from build123d import *

# Parameters (mm, degrees)
SKETCH1_W           = 70
SKETCH1_H           = 70
SKETCH1_R           = 1.65
BOSS_EXTRUDE1_DEPTH = 6.35
CUT_EXTRUDE1_REACH  = 51.903
SKETCH2_R           = 1.1
CUT_EXTRUDE2_REACH  = 51.903
SKETCH3_R           = 9.65
CUT_EXTRUDE3_REACH  = 51.903
SKETCH4_R           = 2.1
SKETCH5_R           = 4.5
CUT_EXTRUDE4_DEPTH  = 2.5


with BuildPart() as part:
    # Sketch1 → Boss-Extrude1 (new body)
    with BuildSketch(Plane(origin=(0, 0, 0), x_dir=(1, 0, 0), z_dir=(0, 1, 0))):
        Rectangle(SKETCH1_W, SKETCH1_H)
        with Locations(Location((0, 13, 0), (0, 0, 270))):
            Circle(SKETCH1_R, mode=Mode.SUBTRACT)
        with Locations(Location((13, 0, 0), (0, 0, 270))):
            Circle(SKETCH1_R, mode=Mode.SUBTRACT)
        with Locations(Location((0, -13, 0), (0, 0, 270))):
            Circle(SKETCH1_R, mode=Mode.SUBTRACT)
        with Locations(Location((-13, 0, 0), (0, 0, 270))):
            Circle(SKETCH1_R, mode=Mode.SUBTRACT)
    extrude(amount=BOSS_EXTRUDE1_DEPTH)

    # Sketch2 → Cut-Extrude1 (cut, up to next)
    with BuildSketch(Plane(origin=(0, 6.35, 0), x_dir=(1, 0, 0), z_dir=(0, 1, 0)), mode=Mode.PRIVATE) as cut_extrude1_sk1:
        with Locations(Location((16.375, 28, 0), (0, 0, 270))):
            Circle(SKETCH2_R)
    cut_extrude1_tool1 = extrude(cut_extrude1_sk1.sketch, amount=-CUT_EXTRUDE1_REACH, mode=Mode.PRIVATE) & part.part
    # Sketch2 → Cut-Extrude1 (cut, up to next)
    with BuildSketch(Plane(origin=(0, 6.35, 0), x_dir=(1, 0, 0), z_dir=(0, 1, 0)), mode=Mode.PRIVATE) as cut_extrude1_sk2:
        with Locations(Location((28.375, 28, 0), (0, 0, 270))):
            Circle(SKETCH2_R)
    cut_extrude1_tool2 = extrude(cut_extrude1_sk2.sketch, amount=-CUT_EXTRUDE1_REACH, mode=Mode.PRIVATE) & part.part
    # Sketch2 → Cut-Extrude1 (cut, up to next)
    with BuildSketch(Plane(origin=(0, 6.35, 0), x_dir=(1, 0, 0), z_dir=(0, 1, 0)), mode=Mode.PRIVATE) as cut_extrude1_sk3:
        with Locations(Location((28.375, 20, 0), (0, 0, 270))):
            Circle(SKETCH2_R)
    cut_extrude1_tool3 = extrude(cut_extrude1_sk3.sketch, amount=-CUT_EXTRUDE1_REACH, mode=Mode.PRIVATE) & part.part
    # Sketch2 → Cut-Extrude1 (cut, up to next)
    with BuildSketch(Plane(origin=(0, 6.35, 0), x_dir=(1, 0, 0), z_dir=(0, 1, 0)), mode=Mode.PRIVATE) as cut_extrude1_sk4:
        with Locations(Location((-28.375, 20, 0), (0, 0, 270))):
            Circle(SKETCH2_R)
    cut_extrude1_tool4 = extrude(cut_extrude1_sk4.sketch, amount=-CUT_EXTRUDE1_REACH, mode=Mode.PRIVATE) & part.part
    # Sketch2 → Cut-Extrude1 (cut, up to next)
    with BuildSketch(Plane(origin=(0, 6.35, 0), x_dir=(1, 0, 0), z_dir=(0, 1, 0)), mode=Mode.PRIVATE) as cut_extrude1_sk5:
        with Locations(Location((-28.375, 28, 0), (0, 0, 270))):
            Circle(SKETCH2_R)
    cut_extrude1_tool5 = extrude(cut_extrude1_sk5.sketch, amount=-CUT_EXTRUDE1_REACH, mode=Mode.PRIVATE) & part.part
    # Sketch2 → Cut-Extrude1 (cut, up to next)
    with BuildSketch(Plane(origin=(0, 6.35, 0), x_dir=(1, 0, 0), z_dir=(0, 1, 0)), mode=Mode.PRIVATE) as cut_extrude1_sk6:
        with Locations(Location((-16.375, 28, 0), (0, 0, 270))):
            Circle(SKETCH2_R)
    cut_extrude1_tool6 = extrude(cut_extrude1_sk6.sketch, amount=-CUT_EXTRUDE1_REACH, mode=Mode.PRIVATE) & part.part
    # Sketch2 → Cut-Extrude1 (cut, up to next)
    with BuildSketch(Plane(origin=(0, 6.35, 0), x_dir=(1, 0, 0), z_dir=(0, 1, 0)), mode=Mode.PRIVATE) as cut_extrude1_sk7:
        with Locations(Location((28.375, -20, 0), (0, 0, 270))):
            Circle(SKETCH2_R)
    cut_extrude1_tool7 = extrude(cut_extrude1_sk7.sketch, amount=-CUT_EXTRUDE1_REACH, mode=Mode.PRIVATE) & part.part
    # Sketch2 → Cut-Extrude1 (cut, up to next)
    with BuildSketch(Plane(origin=(0, 6.35, 0), x_dir=(1, 0, 0), z_dir=(0, 1, 0)), mode=Mode.PRIVATE) as cut_extrude1_sk8:
        with Locations(Location((28.375, -28, 0), (0, 0, 270))):
            Circle(SKETCH2_R)
    cut_extrude1_tool8 = extrude(cut_extrude1_sk8.sketch, amount=-CUT_EXTRUDE1_REACH, mode=Mode.PRIVATE) & part.part
    # Sketch2 → Cut-Extrude1 (cut, up to next)
    with BuildSketch(Plane(origin=(0, 6.35, 0), x_dir=(1, 0, 0), z_dir=(0, 1, 0)), mode=Mode.PRIVATE) as cut_extrude1_sk9:
        with Locations(Location((16.375, -28, 0), (0, 0, 270))):
            Circle(SKETCH2_R)
    cut_extrude1_tool9 = extrude(cut_extrude1_sk9.sketch, amount=-CUT_EXTRUDE1_REACH, mode=Mode.PRIVATE) & part.part
    # Sketch2 → Cut-Extrude1 (cut, up to next)
    with BuildSketch(Plane(origin=(0, 6.35, 0), x_dir=(1, 0, 0), z_dir=(0, 1, 0)), mode=Mode.PRIVATE) as cut_extrude1_sk10:
        with Locations(Location((-16.375, -28, 0), (0, 0, 270))):
            Circle(SKETCH2_R)
    cut_extrude1_tool10 = extrude(cut_extrude1_sk10.sketch, amount=-CUT_EXTRUDE1_REACH, mode=Mode.PRIVATE) & part.part
    # Sketch2 → Cut-Extrude1 (cut, up to next)
    with BuildSketch(Plane(origin=(0, 6.35, 0), x_dir=(1, 0, 0), z_dir=(0, 1, 0)), mode=Mode.PRIVATE) as cut_extrude1_sk11:
        with Locations(Location((-28.375, -20, 0), (0, 0, 270))):
            Circle(SKETCH2_R)
    cut_extrude1_tool11 = extrude(cut_extrude1_sk11.sketch, amount=-CUT_EXTRUDE1_REACH, mode=Mode.PRIVATE) & part.part
    # Sketch2 → Cut-Extrude1 (cut, up to next)
    with BuildSketch(Plane(origin=(0, 6.35, 0), x_dir=(1, 0, 0), z_dir=(0, 1, 0)), mode=Mode.PRIVATE) as cut_extrude1_sk12:
        with Locations(Location((-28.375, -28, 0), (0, 0, 270))):
            Circle(SKETCH2_R)
    cut_extrude1_tool12 = extrude(cut_extrude1_sk12.sketch, amount=-CUT_EXTRUDE1_REACH, mode=Mode.PRIVATE) & part.part
    add(cut_extrude1_tool1.solids().sort_by_distance((16.375, 6.35, -28))[0], mode=Mode.SUBTRACT)
    add(cut_extrude1_tool2.solids().sort_by_distance((28.375, 6.35, -28))[0], mode=Mode.SUBTRACT)
    add(cut_extrude1_tool3.solids().sort_by_distance((28.375, 6.35, -20))[0], mode=Mode.SUBTRACT)
    add(cut_extrude1_tool4.solids().sort_by_distance((-28.375, 6.35, -20))[0], mode=Mode.SUBTRACT)
    add(cut_extrude1_tool5.solids().sort_by_distance((-28.375, 6.35, -28))[0], mode=Mode.SUBTRACT)
    add(cut_extrude1_tool6.solids().sort_by_distance((-16.375, 6.35, -28))[0], mode=Mode.SUBTRACT)
    add(cut_extrude1_tool7.solids().sort_by_distance((28.375, 6.35, 20))[0], mode=Mode.SUBTRACT)
    add(cut_extrude1_tool8.solids().sort_by_distance((28.375, 6.35, 28))[0], mode=Mode.SUBTRACT)
    add(cut_extrude1_tool9.solids().sort_by_distance((16.375, 6.35, 28))[0], mode=Mode.SUBTRACT)
    add(cut_extrude1_tool10.solids().sort_by_distance((-16.375, 6.35, 28))[0], mode=Mode.SUBTRACT)
    add(cut_extrude1_tool11.solids().sort_by_distance((-28.375, 6.35, 20))[0], mode=Mode.SUBTRACT)
    add(cut_extrude1_tool12.solids().sort_by_distance((-28.375, 6.35, 28))[0], mode=Mode.SUBTRACT)

    # Sketch3 → Cut-Extrude2 (cut, up to next)
    with BuildSketch(Plane(origin=(0, 6.35, 0), x_dir=(1, 0, 0), z_dir=(0, 1, 0)), mode=Mode.PRIVATE) as cut_extrude2_sk1:
        with Locations(Location((0, 0, 0), (0, 0, 270))):
            Circle(SKETCH3_R)
    cut_extrude2_tool1 = extrude(cut_extrude2_sk1.sketch, amount=-CUT_EXTRUDE2_REACH, mode=Mode.PRIVATE) & part.part
    add(cut_extrude2_tool1.solids().sort_by_distance((0, 6.35, 0))[0], mode=Mode.SUBTRACT)

    # Sketch4 → Cut-Extrude3 (cut, up to next)
    with BuildSketch(Plane(origin=(0, 6.35, 0), x_dir=(1, 0, 0), z_dir=(0, 1, 0)), mode=Mode.PRIVATE) as cut_extrude3_sk1:
        with Locations(Location((0, 27.5, 0), (0, 0, 270))):
            Circle(SKETCH4_R)
    cut_extrude3_tool1 = extrude(cut_extrude3_sk1.sketch, amount=-CUT_EXTRUDE3_REACH, mode=Mode.PRIVATE) & part.part
    # Sketch4 → Cut-Extrude3 (cut, up to next)
    with BuildSketch(Plane(origin=(0, 6.35, 0), x_dir=(1, 0, 0), z_dir=(0, 1, 0)), mode=Mode.PRIVATE) as cut_extrude3_sk2:
        with Locations(Location((27.5, 0, 0), (0, 0, 270))):
            Circle(SKETCH4_R)
    cut_extrude3_tool2 = extrude(cut_extrude3_sk2.sketch, amount=-CUT_EXTRUDE3_REACH, mode=Mode.PRIVATE) & part.part
    # Sketch4 → Cut-Extrude3 (cut, up to next)
    with BuildSketch(Plane(origin=(0, 6.35, 0), x_dir=(1, 0, 0), z_dir=(0, 1, 0)), mode=Mode.PRIVATE) as cut_extrude3_sk3:
        with Locations(Location((0, -27.5, 0), (0, 0, 270))):
            Circle(SKETCH4_R)
    cut_extrude3_tool3 = extrude(cut_extrude3_sk3.sketch, amount=-CUT_EXTRUDE3_REACH, mode=Mode.PRIVATE) & part.part
    # Sketch4 → Cut-Extrude3 (cut, up to next)
    with BuildSketch(Plane(origin=(0, 6.35, 0), x_dir=(1, 0, 0), z_dir=(0, 1, 0)), mode=Mode.PRIVATE) as cut_extrude3_sk4:
        with Locations(Location((-27.5, 0, 0), (0, 0, 270))):
            Circle(SKETCH4_R)
    cut_extrude3_tool4 = extrude(cut_extrude3_sk4.sketch, amount=-CUT_EXTRUDE3_REACH, mode=Mode.PRIVATE) & part.part
    add(cut_extrude3_tool1.solids().sort_by_distance((0, 6.35, -27.5))[0], mode=Mode.SUBTRACT)
    add(cut_extrude3_tool2.solids().sort_by_distance((27.5, 6.35, 0))[0], mode=Mode.SUBTRACT)
    add(cut_extrude3_tool3.solids().sort_by_distance((0, 6.35, 27.5))[0], mode=Mode.SUBTRACT)
    add(cut_extrude3_tool4.solids().sort_by_distance((-27.5, 6.35, 0))[0], mode=Mode.SUBTRACT)

    # Sketch5 → Cut-Extrude4 (cut)
    with BuildSketch(Plane(origin=(0, 6.35, 0), x_dir=(1, 0, 0), z_dir=(0, 1, 0))):
        with Locations(Location((0, 27.5, 0), (0, 0, 270))):
            Circle(SKETCH5_R)
        with Locations(Location((27.5, 0, 0), (0, 0, 270))):
            Circle(SKETCH5_R)
        with Locations(Location((0, -27.5, 0), (0, 0, 270))):
            Circle(SKETCH5_R)
        with Locations(Location((-27.5, 0, 0), (0, 0, 270))):
            Circle(SKETCH5_R)
    extrude(amount=-CUT_EXTRUDE4_DEPTH, mode=Mode.SUBTRACT)


solid = part.part
Build history of the part. All positions in model axes, mm. A direction names the side the tool comes from. Round coordinates to 2 decimals unless told otherwise and drop trailing zeros. Loops run counter-clockwise (first coordinate to the right, second up) from the corner with the lowest first, then second, coordinate; pieces in that order, holes last. Notation, with made-up numbers: (68, 40.5) -> (93, 40.5) arc R10 ccw to (93, 48.5) -> close; hole circle Ø1 at (38, 2). An arc over 180 degrees is marked (long way). One line per item, written item: value. Start each with the question number.
Q1. Drop flat-ended pins along their axis: pin 1 Ø2.5 at (x, z) = (0, -13) entering from -Y; pin 2 Ø2.5 at (x, z) = (1, -27.5) entering from +Y. Give the stop position or say it passes through.
Q2. Cut at C-C on y = 2. Count the separate pieces of the cut face and the enclosed holes in it, plus the area to 3 significant figures.
Q3. Cut at B-B on z = -13. List the corners of the cut face in (x, y), plus the area to 3 significant figures.
Q4. Cut at D-D on z = -28. List the corners of the cut face in (x, y) (3 decimals).
Q5. 3-axis set-ups, long thin cutter, end or side, ignore diameter. For faces 1 (the face through (9.568, 3.219, -1.256)), 2 (the face through (29, 3.85, 2)): which of +Z, -Z, +X, -X, +Y, -Y reach the whole face in a straight line?
Q6. Two-plate mould, pull along Z, no slides. Class faces 3 (the face through (0, 3, 35)), 4 (the face through (-17.45, 3.22, -28.24)), 5 (the face through (35, 3, 0)): released by +Z, released by -Z, zero draft, split by the parting line, or undercut.
Q7. Probe line 1 along X through (y, z) = (4.25, 20) (3 decimals); line 2 along X through (y, z) = (4.5, -1); line 3 along X through (y, z) = (6, -2). List the from-to ranges inside material, lowest first.
Q8. Cut at A-A on z = 20. List the corners of the cut face in (x, y) (3 decimals).
Computed:
1. pin 1: through
1. pin 2: y = 3.85
2. separate pieces: 1
2. enclosed holes: 21
2. area: 4,470 mm²
3. outline: (-35, 0) -> (-1.65, 0) -> (-1.65, 6.35) -> (-35, 6.35) -> close; (1.65, 0) -> (35, 0) -> (35, 6.35) -> (1.65, 6.35) -> close
3. area: 424 mm²
4. outline: (-35, 0) -> (-29.475, 0) -> (-29.475, 6.35) -> (-35, 6.35) -> close; (-27.275, 0) -> (-17.475, 0) -> (-17.475, 6.35) -> (-27.275, 6.35) -> close; (-15.275, 0) -> (-2.04, 0) -> (-2.04, 3.85) -> (-4.472, 3.85) -> (-4.472, 6.35) -> (-15.275, 6.35) -> close; (2.04, 0) -> (15.275, 0) -> (15.275, 6.35) -> (4.472, 6.35) -> (4.472, 3.85) -> (2.04, 3.85) -> close; (17.475, 0) -> (27.275, 0) -> (27.275, 6.35) -> (17.475, 6.35) -> close; (29.475, 0) -> (35, 0) -> (35, 6.35) -> (29.475, 6.35) -> close
5. face 1: +Y, -Y
5. face 2: +Y
6. face 3: released by +Z
6. face 4: undercut
6. face 5: zero draft
7. line 1: -35 to -29.475, -27.275 to 27.275, 29.475 to 35
7. line 2: -35 to -31.89, -23.11 to -14.31, -11.69 to -9.6, 9.6 to 11.69, 14.31 to 23.11, 31.89 to 35
7. line 3: -35 to -31.53, -23.47 to -9.44, 9.44 to 23.47, 31.53 to 35
8. outline: (-35, 0) -> (-29.475, 0) -> (-29.475, 6.35) -> (-35, 6.35) -> close; (-27.275, 0) -> (27.275, 0) -> (27.275, 6.35) -> (-27.275, 6.35) -> close; (29.475, 0) -> (35, 0) -> (35, 6.35) -> (29.475, 6.35) -> close
